The model under review builds one solid part; all positions refer to its coordinate system, in mm. Face numbers are marked on the shaded views. A direction names the side the tool comes from. Give positions to 0.01 mm unless a question says otherwise; leave off trailing zeros. Loops run counter-clockwise (first coordinate to the right, second up) from the corner with the lowest first, then second, coordinate; pieces in that order, holes last. Notation, with made-up numbers: M 37.25,63 L 74.25,63 A4 ccw 74.25,68 Z; hole C -26,-39 d10. An arc over 180 degrees is marked long. Return JSON: item names as keys, results as strings.
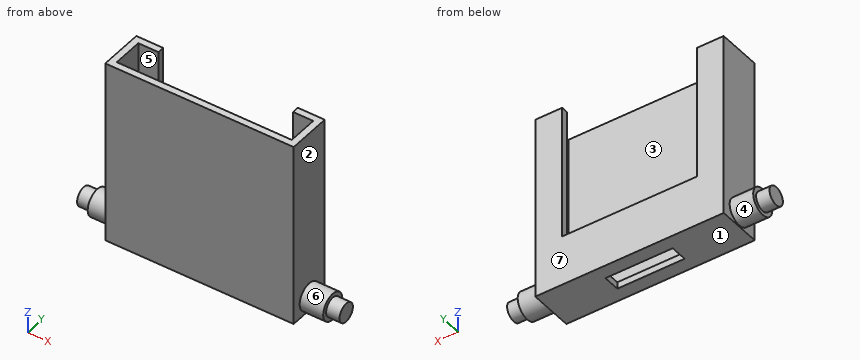
```python
from build123d import *

# Parameters (mm, degrees)
SKETCH1_W           = 71.12
SKETCH1_H           = 69.85
BOSS_EXTRUDE1_DEPTH = 16.51
SHELL1_T            = -2.54
SKETCH4_R           = 5.08
BOSS_EXTRUDE2_DEPTH = 8.89
BOSS_EXTRUDE3_START = 8.89
SKETCH3_R           = 5.08
BOSS_EXTRUDE3_DEPTH = 8.89
SKETCH6_R           = 3.556
BOSS_EXTRUDE4_DEPTH = 5.08
BOSS_EXTRUDE5_START = 5.08
SKETCH5_R           = 3.556
BOSS_EXTRUDE5_DEPTH = 5.08
SKETCH7_W           = 50.8
SKETCH7_H           = 50.8
CUT_EXTRUDE1_DEPTH  = 2.54
SKETCH8_W           = 25.4
SKETCH8_H           = 6.35
CUT_EXTRUDE2_DEPTH  = 2.54


with BuildPart() as part:
    # Sketch1 → Boss-Extrude1 (new body)
    with BuildSketch(Plane(origin=(0, 0, 0), x_dir=(1, 0, 0), z_dir=(0, 1, 0))):
        Rectangle(SKETCH1_W, SKETCH1_H)
    extrude(amount=BOSS_EXTRUDE1_DEPTH)

    # Shell1
    shell1_openings = [part.faces().sort_by_distance(p)[0] for p in [
        (0, 8.255, 34.925),
    ]]
    offset(amount=SHELL1_T, openings=shell1_openings, kind=Kind.INTERSECTION)

    # Sketch4 → Boss-Extrude2 (add)
    with BuildSketch(Plane.ZY.offset(35.56)):
        with Locations(Location((-29.337, 8.255, 0), (0, 0, 180))):
            Circle(SKETCH4_R)
    extrude(amount=BOSS_EXTRUDE2_DEPTH)

    # Sketch3 → Boss-Extrude3 (add)
    with BuildSketch(Plane(origin=(35.56, 0, 0), x_dir=(0, 0, -1), z_dir=(1, 0, 0)).offset(BOSS_EXTRUDE3_START)):
        with Locations((29.337, 8.255)):
            Circle(SKETCH3_R)
    extrude(amount=-BOSS_EXTRUDE3_DEPTH)

    # Sketch6 → Boss-Extrude4 (add)
    with BuildSketch(Plane(origin=(44.45, 0, 0), x_dir=(0, 0, -1), z_dir=(1, 0, 0))):
        with Locations((29.337, 8.255)):
            Circle(SKETCH6_R)
    extrude(amount=BOSS_EXTRUDE4_DEPTH)

    # Sketch5 → Boss-Extrude5 (add)
    with BuildSketch(Plane.ZY.offset(44.45).offset(BOSS_EXTRUDE5_START)):
        with Locations(Location((-29.337, 8.255, 0), (0, 0, 180))):
            Circle(SKETCH5_R)
    extrude(amount=-BOSS_EXTRUDE5_DEPTH)

    # Sketch7 → Cut-Extrude1 (cut)
    with BuildSketch(Plane(origin=(0, 16.51, 0), x_dir=(1, 0, 0), z_dir=(0, 1, 0))):
        with Locations((0, -9.525)):
            Rectangle(SKETCH7_W, SKETCH7_H)
    extrude(amount=-CUT_EXTRUDE1_DEPTH, mode=Mode.SUBTRACT)

    # Sketch8 → Cut-Extrude2 (cut)
    with BuildSketch(Plane(origin=(0, 0, -34.925), x_dir=(-1, 0, 0), z_dir=(0, 0, -1))):
        with Locations((0, 8.255)):
            Rectangle(SKETCH8_W, SKETCH8_H)
    extrude(amount=-CUT_EXTRUDE2_DEPTH, mode=Mode.SUBTRACT)


solid = part.part
```
1) Consider section A-A on x = 30. Write out the cut boundary in (y, z) (3 decimals), then the cut area to 3 significant figures.
From the geometry:
{"outline": "M 0,-34.925 L 16.51,-34.925 L 16.51,34.925 L 13.97,34.925 L 13.97,-32.385 L 2.54,-32.385 L 2.54,34.925 L 0,34.925 Z", "area": "384 mm²"}
2) Insertion check: pin 1 (3 mm diameter, centred on x = -8.5, y = 6.5, fed in from +Z) (3 decimals); pin 2 (1.5 mm diameter, centred on y = 2.5, z = -1, fed in from -X); pin 3 (1.3 mm diameter, centred on y = 15.5, z = 11, fed in from +X). Each pin has a flat end and moves straight along its axis. Give the tip position at first contact, or say it passes through.
From the geometry:
{"pin 1": "z = -32.385", "pin 2": "x = -35.56", "pin 3": "x = 35.56"}
3) The part is to be moulded in two halves that separate along X. For the marked faces 1, 2 and 3, say which applies: released by +X, released by -X, zero draft, split by the parting line, or undercut.
From the geometry:
{"face 1": "zero draft", "face 2": "released by +X", "face 3": "undercut"}
4) Tool access review of the marked faces 4, 5, 6 and 7: name each direction out of +Z, -Z, +X, -X, +Y, -Y from which nothing blocks a thin tool from reaching the whole face with its end or side.
From the geometry:
{"face 4": "-X", "face 5": "+Z", "face 6": "+X", "face 7": "+Z, -Z, +X, -X, +Y"}
5) Wall thickness on L1, parallel to X at y = 12.5, z = 8.5; L2, parallel to Y at x = 27, z = -11; L3, parallel to X at y = 15.25, z = -12.5: over which ranges is each line inside the solid? List them lowest first. Write a range as from..to.
From the geometry:
{"L1": "-35.56..-33.02, 33.02..35.56", "L2": "0..2.54, 13.97..16.51", "L3": "-35.56..-25.4, 25.4..35.56"}
6) Consider section B-B on y = 9.75. Write out the cut boundary in (x, z) (3 decimals).
From the geometry:
{"outline": "M -49.53,-32.563 L -44.45,-32.563 L -44.45,-34.192 L -35.56,-34.192 L -35.56,-34.925 L -12.7,-34.925 L -12.7,-32.385 L -33.02,-32.385 L -33.02,34.925 L -35.56,34.925 L -35.56,-24.482 L -44.45,-24.482 L -44.45,-26.111 L -49.53,-26.111 Z; M 12.7,-34.925 L 35.56,-34.925 L 35.56,-34.192 L 44.45,-34.192 L 44.45,-32.563 L 49.53,-32.563 L 49.53,-26.111 L 44.45,-26.111 L 44.45,-24.482 L 35.56,-24.482 L 35.56,34.925 L 33.02,34.925 L 33.02,-32.385 L 12.7,-32.385 Z"}
7) Consider section C-C on z = -7.5. Write out the cut boundary in (x, y), then the cut area to 3 significant figures.
From the geometry:
{"outline": "M -35.56,0 L 35.56,0 L 35.56,16.51 L 25.4,16.51 L 25.4,13.97 L 33.02,13.97 L 33.02,2.54 L -33.02,2.54 L -33.02,13.97 L -25.4,13.97 L -25.4,16.51 L -35.56,16.51 Z", "area": "290 mm²"}
8) Consider section D-D on z = -28. Write out the cut boundary in (x, y).
From the geometry:
{"outline": "M -49.53,4.96 L -44.45,4.96 L -44.45,3.35 L -35.56,3.35 L -35.56,0 L 35.56,0 L 35.56,3.35 L 44.45,3.35 L 44.45,4.96 L 49.53,4.96 L 49.53,11.55 L 44.45,11.55 L 44.45,13.16 L 35.56,13.16 L 35.56,16.51 L -35.56,16.51 L -35.56,13.16 L -44.45,13.16 L -44.45,11.55 L -49.53,11.55 Z; hole M -33.02,2.54 L 33.02,2.54 L 33.02,13.97 L -33.02,13.97 Z"}
